Part model, mm, in its own coordinate system. Face numbers are marked on the shaded views. A direction names the side the tool comes from. Round coordinates to 2 decimals unless told otherwise and drop trailing zeros. Order: outer loops, then holes, each group sorted by start corner. A loop starts at its lowest first (then second) coordinate and runs counter-clockwise, first axis right, second up. Notation, with made-up numbers: (19.25, 44) -> (72.25, 44) arc R28 cw to (72.25, 63) -> close; hole circle Ø4 at (28.5, 69). An arc over 180 degrees is marked (long way). Answer as a JSON object with one key per item and string values. Group by question number.
```python
from build123d import *

# Parameters (mm, degrees)
F1_DEPTH = 60
F2_SIZE  = 5
F3_R     = 25
F4_DEPTH = 25


with BuildPart() as f1:
    # F0 (on Front) → F1 (new body)
    with BuildSketch(Plane.XZ):
        with BuildLine():
            Line((32.580328, 24.762304), (-22.035015, 24.762304))
            ThreePointArc((-22.035015, 24.762304), (-39.712685, 17.439974), (-47.035015, -0.237696))
            Line((-47.035015, -0.237696), (-47.035015, -75.237696))
            Line((-47.035015, -75.237696), (27.964985, -75.237696))
            ThreePointArc((27.964985, -75.237696), (45.642654, -67.915365), (52.964985, -50.237696))
            Line((52.964985, -50.237696), (52.964985, 0))
            Line((52.964985, 0), (34.512423, 22.415288))
            Line((34.512423, 22.415288), (32.580328, 24.762304))
        make_face()
    extrude(amount=F1_DEPTH)

    # F2
    f2_edges = [f1.edges().sort_by_distance(p)[0] for p in [
        (-39.712685, -60, 17.439974),
        (5.272656, -60, 24.762304),
        (42.772656, -60, 12.381152),
        (52.964985, -60, -25.118848),
        (45.642654, -60, -67.915365),
        (-9.535015, -60, -75.237696),
        (-47.035015, -60, -37.737696),
        (-39.712685, 0, 17.439974),
        (5.272656, 0, 24.762304),
        (42.772656, 0, 12.381152),
        (45.642654, 0, -67.915365),
        (-9.535015, 0, -75.237696),
    ]]
    chamfer(f2_edges, length=F2_SIZE)

    # F3 (on face) → F4 (cut)
    with BuildSketch(Plane.XZ.offset(60)):
        with Locations((0, -30.696294)):
            Circle(F3_R)
    extrude(amount=-F4_DEPTH, mode=Mode.SUBTRACT)


solid = f1.part
```
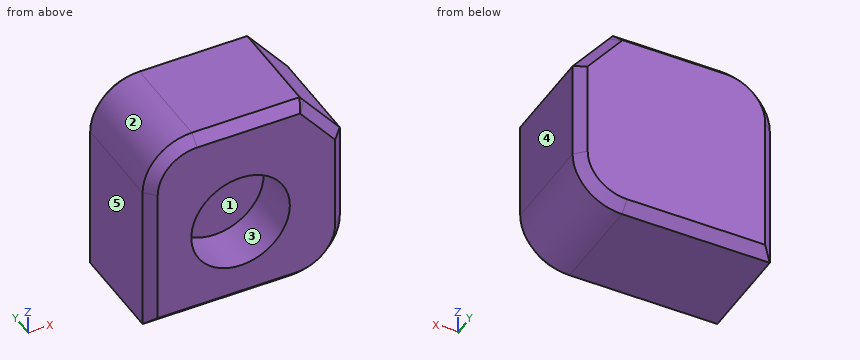
Q1. Band-saw the part on A-A (y = -22.5). List the corners of the cut face in (x, z).
Q2. Which spindle directions (+Z, -Z, +X, -X, +Y, -Y) get a long thin tool onto all of the face, cutting with end or side? Do the marked faces 1 and 2. Say none if no direction does.
Q3. Band-saw the part on B-B (x = 0). List the corners of the cut face in (y, z), plus the area to 3 significant figures.
Q4. Wall check: line 1 (Z direction, x = 0, y = -49.75); line 2 (Y direction, x = -5, z = -16); line 3 (X direction, y = -39, z = -34). Give the ranges that are in metal, low to high. Write a range as [from, to].
Q5. Drop flat-ended pins along their axis: pin 1 Ø15 at (x, z) = (-5.5, -28.5) entering from -Y; pin 2 Ø3 at (x, y) = (30, -8.5) entering from -Z; pin 3 Ø6 at (x, y) = (42, -21.5) entering from +Z. Give the stop position or say it passes through.
Q6. Band-saw the part on C-C (z = -28.5). List the corners of the cut face in (x, y), plus the area to 3 significant figures.
Q7. Two-plate mould, pull along X, no slides. Class the marked faces 3, 4 and 5: +X half, -X half, draft (parallel to the pull), parting line (faces both ways), or undercut.
Completed:
{
 "1": {"outline": "(-47.04, -75.24) -> (27.96, -75.24) arc R25 ccw to (52.96, -50.24) -> (52.96, 0) -> (32.58, 24.76) -> (-22.04, 24.76) arc R25 ccw to (-47.04, -0.24) -> close"},
 "2": {"face 1": "-Y", "face 2": "+Z, -X, +Y, -Y"},
 "3": {"outline": "(-60, -70.24) -> (-55, -75.24) -> (-5, -75.24) -> (0, -70.24) -> (0, 19.76) -> (-5, 24.76) -> (-55, 24.76) -> (-60, 19.76) -> (-60, -5.7) -> (-35, -5.7) -> (-35, -55.7) -> (-60, -55.7) -> close", "area": "4,700 mm2"},
 "4": {"line 1": "[-75.24, -55.7], [-5.7, 24.76]", "line 2": "[-35, 0]", "line 3": "[-47.04, -24.78], [24.78, 52.96]"},
 "5": {"pin 1": "y = -35", "pin 2": "z = -75.23", "pin 3": "z = 16.96"},
 "6": {"outline": "(-47.04, -55) -> (-42.04, -60) -> (-24.9, -60) -> (-24.9, -35) -> (24.9, -35) -> (24.9, -60) -> (47.96, -60) -> (52.96, -55) -> (52.96, -5) -> (47.96, 0) -> (-42.04, 0) -> (-47.04, -5) -> close", "area": "4,700 mm2"},
 "7": {"face 3": "undercut", "face 4": "+X half", "face 5": "-X half"}
}
